Part print with two shaded views. Sizes in mm from the minimum x, y, z corner. A direction names the side the tool comes from. Round coordinates to 2 decimals unless told otherwise and drop trailing zeros. Order: outer loops, then holes, each group sorted by start corner. A loop starts at its lowest first (then second) coordinate and runs counter-clockwise, first axis right, second up. Notation, with made-up numbers: (-11, 48) - (27, 48) arc R26 cw to (27, 75) - close; hole circle Ø11 at (-28.5, 4.25). An arc over 180 degrees is marked (long way). Answer as CSV lines item,"result". Start each with the question number.
1. Band-saw the part on A-A on y = 5. List the corners of the cut face in (x, z), then the cut area to 3 significant figures.
2. Wall check: line 1 along Z through (x, y) = (12, 5.25); line 2 along Y through (x, z) = (36, 7); line 3 along Y through (x, z) = (34, 4). Give the ranges that are in metal, low to high. Write a range as [from, to].
3. Band-saw the part on C-C on z = 12. List the corners of the cut face in (x, y), then the cut area to 3 significant figures.
4. Pull direction Y, two halves, no side cores. Call the marked faces 4, 5 and 6: released by +Y, released by -Y, zero draft, split by the parting line, or undercut.
5. Band-saw the part on B-B on z = 4. List the corners of the cut face in (x, y), then the cut area to 3 significant figures.
6. Band-saw the part on D-D on y = 35. List the corners of the cut face in (x, z), then the cut area to 4 significant figures.
7. 3-axis set-ups, long thin cutter, end or side, ignore diameter. For the marked faces 1, 2 and 3: which of +Z, -Z, +X, -X, +Y, -Y reach the whole face in a straight line?
8. Pin check, flat tips, straight feed: pin 1 Ø6.5 at (y, z) = (50.5, 8) entering from -X; pin 2 Ø6 at (y, z) = (17, 10.5) entering from +X; pin 3 Ø17.5 at (y, z) = (35, 28.5) entering from -X. Stop position of each tip, or through.
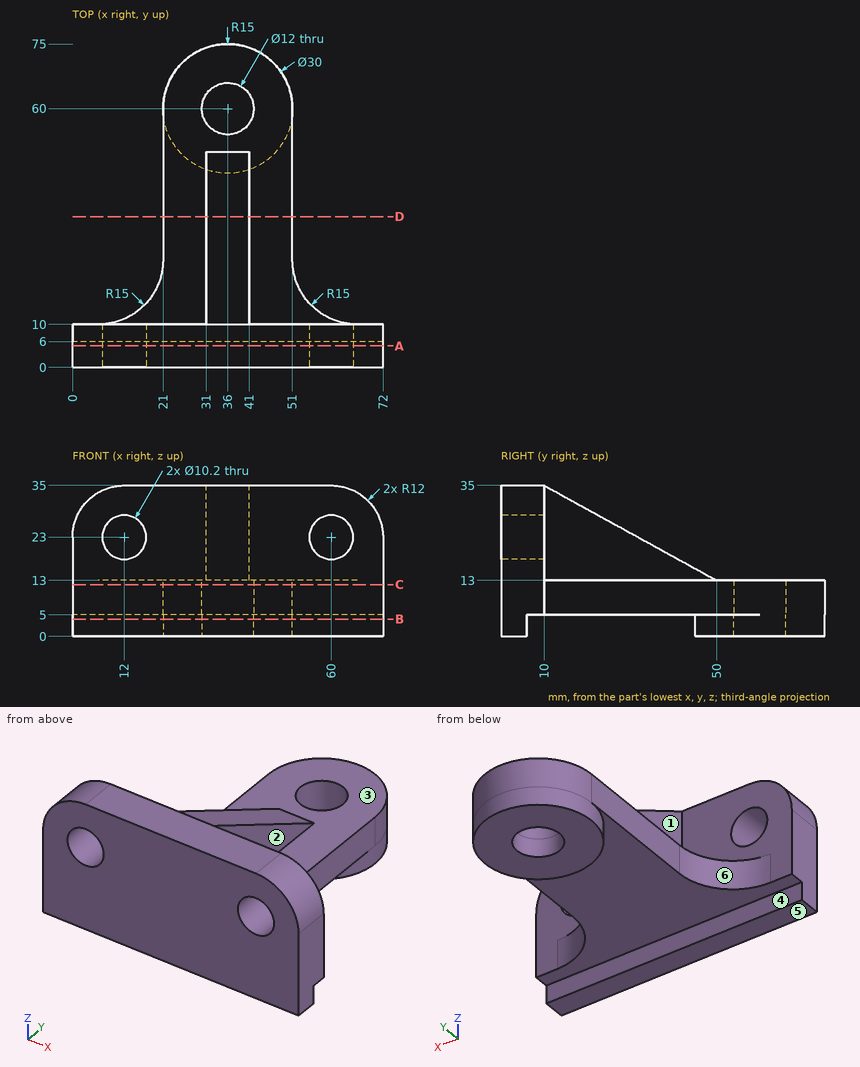
Reply:
1,outline,"(0, 0) - (72, 0) - (72, 23) arc R12 ccw to (60, 35) - (12, 35) arc R12 ccw to (0, 23) - close; hole circle Ø10.2 at (12, 23); hole circle Ø10.2 at (60, 23)"
1,area,"2,290 mm2"
2,line 1,"z = [0, 17.9], [28.1, 35]"
2,line 2,"y = [0, 54], [66, 75]"
2,line 3,"y = [0, 6], [45.13, 54.34], [65.66, 74.87]"
3,outline,"(0, 0) - (72, 0) - (72, 10) - (66, 10) arc R15 cw to (51, 25) - (51, 60) arc R15 ccw to (21, 60) - (21, 25) arc R15 cw to (6, 10) - (0, 10) - close; hole circle Ø12 at (36, 60)"
3,area,"2,560 mm2"
4,face 4,"undercut"
4,face 5,"zero draft"
4,face 6,"released by +Y"
5,outline,"(0, 0) - (72, 0) - (72, 6) - (0, 6) - close; circle Ø30 at (36, 60); hole circle Ø12 at (36, 60)"
5,area,"1,030 mm2"
6,outline,"(21, 5) - (51, 5) - (51, 13) - (41, 13) - (41, 21.25) - (31, 21.25) - (31, 13) - (21, 13) - close"
6,area,"322.5 mm2"
7,face 1,"+Z, -X, +Y"
7,face 2,"+Z, +X, +Y"
7,face 3,"+Z, +Y"
8,pin 1,"stops at x = 21"
8,pin 2,"stops at x = 55.8"
8,pin 3,"stops at x = 31"
